from build123d import *

# Parameters (mm, degrees)
SKETCH1_R                  = 12.5
SHAFT_D25X68_DEPTH         = 68
SKETCH2_R                  = 17.5
COLLAR_D35X4_DEPTH         = 4
SKETCH3_R                  = 15
GEARD_SEAT_D30X15_DEPTH    = 15
SKETCH4_W                  = 32
SKETCH4_H                  = 3.5
DOUBLE_FLAT_CUT_25MM_DEPTH = 15
SKETCH5_W                  = 1
SKETCH5_H                  = 2


with BuildPart() as part:
    # Sketch1 → Shaft_D25x68 (new body)
    with BuildSketch(Plane.XY):
        Circle(SKETCH1_R)
    extrude(amount=SHAFT_D25X68_DEPTH)

    # Sketch2 → Collar_D35x4 (add)
    with BuildSketch(Plane.XY.offset(68)):
        Circle(SKETCH2_R)
    extrude(amount=COLLAR_D35X4_DEPTH)

    # Sketch3 → GearD_Seat_D30x15 (add)
    with BuildSketch(Plane.XY.offset(72)):
        Circle(SKETCH3_R)
    extrude(amount=GEARD_SEAT_D30X15_DEPTH)

    # Sketch4 → Double_Flat_Cut_25mm (cut)
    with BuildSketch(Plane.XY.offset(72)):
        with Locations((0, 14.25)):
            Rectangle(SKETCH4_W, SKETCH4_H)
        with Locations((0, -14.25)):
            Rectangle(SKETCH4_W, SKETCH4_H)
    extrude(amount=DOUBLE_FLAT_CUT_25MM_DEPTH, mode=Mode.SUBTRACT)

    # Sketch5 → SnapRing_Groove_D23x1 (revolve, cut)
    with BuildSketch(Plane(origin=(0, 0, 0), x_dir=(0, 0, -1), z_dir=(1, 0, 0)), mode=Mode.PRIVATE) as snapring_groove_d23x1_sk:
        with Locations((-65.5, 12.5)):
            Rectangle(SKETCH5_W, SKETCH5_H)
    revolve(snapring_groove_d23x1_sk.sketch.rotate(Axis((0, 0, 90), (0, 0, -1)), 90), axis=Axis((0, 0, 90), (0, 0, -1)), mode=Mode.SUBTRACT)


solid = part.part
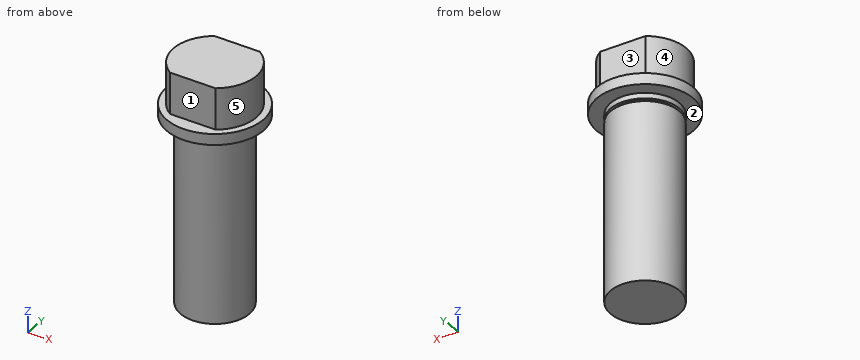
Part model, mm, in its own coordinate system. Face numbers are marked on the shaded views. A direction names the side the tool comes from. Coordinates: 2 decimals unless noted, no trailing zeros. Write each loop counter-clockwise with the first axis right and the second up, starting at its lowest first coordinate (ties: lowest second). Pieces come first, ordered by that corner, then holes. Notation, with made-up numbers: M 69.5,69 L 90.5,69 A13 cw 90.5,74 Z; hole C 32.5,-16 d6. An arc over 180 degrees is marked long. Return JSON: item names as keys, results as strings.
1. Saw through at C-C, the plane z = 70. Write the cut outline in (x, y).
Determined:
{"outline": "C 0,0 d35"}
2. Saw through at B-B, the plane x = -5.5. Write the cut outline in (y, z).
Determined:
{"outline": "M -16.61,68 L -11.22,68 L -11.22,66 L -10.1,66 L -10.1,65 L -11.22,65 L -11.22,0 L 11.22,0 L 11.22,65 L 10.1,65 L 10.1,66 L 11.22,66 L 11.22,68 L 16.61,68 L 16.61,72 L 12.5,72 L 12.5,87 L -12.5,87 L -12.5,72 L -16.61,72 Z"}
3. Saw through at D-D, the plane z = 28.5. Write the cut outline in (x, y), then the cut area to 3 significant figures.
Determined:
{"outline": "C 0,0 d25", "area": "491 mm²"}
4. Flat gauge pins, fed straight in: pin 1 Ø4.5 at (x, z) = (2.5, 76.5) entering from -Y; pin 2 Ø1.5 at (x, z) = (-3.5, 38) entering from +Y; pin 3 Ø8 at (x, z) = (-14, 78) entering from -Y. Where does each tip first touch, or does it go through?
Determined:
{"pin 1": "y = -12.5", "pin 2": "y = 12.19", "pin 3": "y = -11.18"}
5. Probe L1, parallel to Z at x = 10.5, y = -6; L2, parallel to Y at x = 0.5, z = 51; L3, parallel to Z at x = 11, y = -13. List the from-to ranges inside material, lowest first.
Determined:
{"L1": "0 to 65, 66 to 87", "L2": "-12.49 to 12.49", "L3": "68 to 72"}
6. 3-axis set-ups, long thin cutter, end or side, ignore diameter. For the marked faces 1, 2, 3, 4 and 5: which of +Z, -Z, +X, -X, +Y, -Y reach the whole face in a straight line?
Determined:
{"face 1": "+Z, +X, -X, -Y", "face 2": "-Z", "face 3": "+Z, +X, -X, +Y", "face 4": "+Z, -X", "face 5": "+Z, +X"}
7. Saw through at A-A, the plane y = 0. Write the cut outline in (x, z).
Determined:
{"outline": "M -17.5,68 L -12.5,68 L -12.5,66 L -11.5,66 L -11.5,65 L -12.5,65 L -12.5,0 L 12.5,0 L 12.5,65 L 11.5,65 L 11.5,66 L 12.5,66 L 12.5,68 L 17.5,68 L 17.5,72 L 15,72 L 15,87 L -15,87 L -15,72 L -17.5,72 Z"}
